Work out the finished part from the listing and answer in its coordinate system (mm). Face numbers are marked on the shaded views. A direction names the side the tool comes from. Coordinates: 2 decimals unless noted, no trailing zeros. Order: outer loops, then holes, each group sorted by start corner. A loop starts at its lowest first (then second) coordinate and runs counter-clockwise, first axis right, second up. Notation, with made-up numbers: (49.5, 8) -> (58.5, 8) arc R28 ccw to (58.5, 42) -> close; hole circle Ø4 at (-8.5, 12.25). An arc over 180 degrees is marked (long way). Write item = value, one per line. Start each with the question number.
Q1. A flat-ended cylindrical pin translates along its axis: pin 1 (3 mm diameter, centred on x = -5.5, y = 1.5, fed in from +Z). Find the tip coordinate at first contact, or state that the pin passes through.
Q2. The part is cut by section D-D, the plane z = 6. Determine the outline of the cut face in (x, y), plus the area to 3 significant figures.
Q3. The part is cut by section A-A, the plane x = 5.5. Determine the outline of the cut face in (y, z).
Q4. Which of the six approach directions +Z, -Z, +X, -X, +Y, -Y give full straight-line access (tool end or side, diameter ignored) to the marked faces 1, 2, 3, 4 and 5?
Q5. The part is cut by section C-C, the plane x = -2. Determine the outline of the cut face in (y, z), plus the area to 3 significant figures.
Q6. Straight lines are drawn through the part: L1, parallel to Z at x = 5.5, y = 0.25; L2, parallel to X at y = -0.6, z = 6; L3, parallel to Z at x = -1.75, y = -2.25. For each, find the intervals that lie inside material, in ascending order. Write a range as from..to.
Q7. The part is cut by section B-B, the plane z = 1.75. Determine the outline of the cut face in (x, y).
```python
from build123d import *

# Parameters (mm, degrees)
SKETCH1_R             = 1.15
BOSS_EXTRUDE1_DEPTH   = 2.6
BOSS_EXTRUDE2_DEPTH   = 4
SKETCH3_W             = 3
SKETCH3_H             = 5.2
BOSS_EXTRUDE3_DEPTH   = 8
BOSS_EXTRUDE4_DEPTH   = 2.6
CHAMFER1_SIZE         = 1
CHAMFER2_SIZE         = 0.75
CHAMFER2_SIZE2        = 1.299038106
CHAMFER2_PART_2_SIZE  = 0.75
CHAMFER2_PART_2_SIZE2 = 1.299038106


with BuildPart() as part:
    # Sketch1 → Boss-Extrude1 (new body, symmetric)
    with BuildSketch(Plane(origin=(0, 0, 0), x_dir=(1, 0, 0), z_dir=(0, 1, 0))):
        Polygon((4, 0), (8, 0), (8, -12), (3, -12), (3, -4), (-8, -4), (-8, 0), (-4, 0), (-4, -2), (4, -2), align=None)
        with Locations((5.5, -6)):
            Circle(SKETCH1_R, mode=Mode.SUBTRACT)
    extrude(amount=BOSS_EXTRUDE1_DEPTH, both=True)

    # Sketch2 → Boss-Extrude2 (add)
    with BuildSketch(Plane.ZY.offset(8)):
        Polygon((-1.5, -1.25), (-1.5, -2.6), (-4.5, -2.6), (-4.5, 2.6), (-1.5, 2.6), (-1.5, 1.25), (0, 1.25), (0, -1.25), align=None)
    boss_extrude2 = extrude(amount=-BOSS_EXTRUDE2_DEPTH)

    # Mirror1: Boss-Extrude2 across plane
    add(boss_extrude2.mirror(Plane(origin=(0, 0, 0), x_dir=(0, 0, 1), z_dir=(1, 0, 0))))

    # Sketch3 → Boss-Extrude3 (add)
    with BuildSketch(Plane(origin=(-4, 0, 0), x_dir=(0, 0, -1), z_dir=(1, 0, 0))):
        with Locations((3, 0)):
            Rectangle(SKETCH3_W, SKETCH3_H)
    extrude(amount=BOSS_EXTRUDE3_DEPTH)

    # Sketch4 → Boss-Extrude4 (add, symmetric)
    with BuildSketch(Plane(origin=(0, 0, 0), x_dir=(1, 0, 0), z_dir=(0, 1, 0))):
        with BuildLine():
            Line((-4, -1), (-4, -2))
            Line((-4, -2), (-3.464101615, -2))
            ThreePointArc((-3.464101615, -2), (-0.63227674, -0.050287843), (2.666666667, -1.01857603))
            ThreePointArc((2.666666667, -1.01857603), (3.372677996, -0.979231367), (3.333333333, -0.273220038))
            ThreePointArc((3.333333333, -0.273220038), (-0.493116, 0.975624243), (-4, -1))
        make_face()
    extrude(amount=BOSS_EXTRUDE4_DEPTH, both=True)

    # Chamfer1
    chamfer1_edges = [part.edges().sort_by_distance(p)[0] for p in [
        (-8, 1.925, 0),
        (8, 1.925, 0),
        (8, 0, 12),
        (3, 0, 12),
        (3, 0, 4),
        (-8, 0, 4),
        (-8, -1.925, 0),
        (0, -2.6, -4.5),
        (0, 2.6, -4.5),
        (-8, 0, -4.5),
        (-8, -2.6, -3),
        (-8, 2.6, -3),
        (8, -1.925, 0),
        (8, 0, -4.5),
        (8, -2.6, -3),
        (8, 2.6, -3),
    ]]
    chamfer(chamfer1_edges, length=CHAMFER1_SIZE)

    # Chamfer2
    chamfer2_edges = [part.edges().sort_by_distance(p)[0] for p in [
        (4.35, -2.6, 6),
    ]]
    chamfer2_side = [part.faces().sort_by_distance(p)[0] for p in [
        (5.5, -2.6, 0.206155281),
    ]]
    chamfer(chamfer2_edges, length=CHAMFER2_SIZE, length2=CHAMFER2_SIZE2, reference=chamfer2_side[0])

    # Chamfer2 part 2
    chamfer2_part_2_edges = [part.edges().sort_by_distance(p)[0] for p in [
        (4.35, 2.6, 6),
    ]]
    chamfer2_part_2_side = [part.faces().sort_by_distance(p)[0] for p in [
        (5.5, 2.6, 0.206155281),
    ]]
    chamfer(chamfer2_part_2_edges, length=CHAMFER2_PART_2_SIZE, length2=CHAMFER2_PART_2_SIZE2, reference=chamfer2_part_2_side[0])


solid = part.part
```
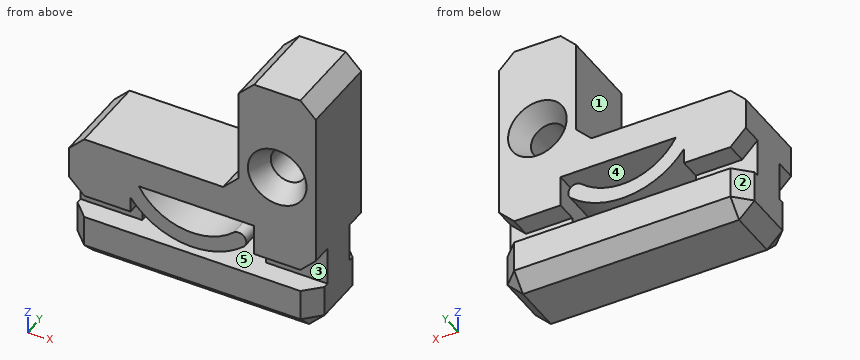
Model answer:
q1.pin_1 = 4
q2.outline = (3, -2.6) -> (3.6, -2.6) -> (4.35, -1.3) -> (4.35, 1.3) -> (3.6, 2.6) -> (3, 2.6) -> close; (6.65, -1.3) -> (7.4, -2.6) -> (8, -2.6) -> (8, 2.6) -> (7.4, 2.6) -> (6.65, 1.3) -> close
q2.area = 12.1 mm2
q3.outline = (-2.6, -3.5) -> (-1.6, -4.5) -> (1.6, -4.5) -> (2.6, -3.5) -> (2.6, -1.5) -> (1.25, -1.5) -> (1.25, 0) -> (2.6, 0) -> (2.6, 4.1) -> (1.3, 4.85) -> (-1.3, 4.85) -> (-2.6, 4.1) -> (-2.6, 0) -> (-1.25, 0) -> (-1.25, -1.5) -> (-2.6, -1.5) -> close; (-2.6, 7.9) -> (-1.3, 7.15) -> (1.3, 7.15) -> (2.6, 7.9) -> (2.6, 12) -> (-2.6, 12) -> close
q4.face_1 = +Z, -X, +Y, -Y
q4.face_2 = -Z, -X, +Y
q4.face_3 = +X, -Y
q4.face_4 = +Y, -Y
q4.face_5 = none
q5.outline = (-2.6, -3.5) -> (-1.6, -4.5) -> (1.6, -4.5) -> (2.6, -3.5) -> (2.6, -1.5) -> (-2.6, -1.5) -> close; (-2.6, -0.58) -> (2.6, -0.58) -> (2.6, 0.54) -> (-2.6, 0.54) -> close; (-2.6, 2) -> (2.6, 2) -> (2.6, 4) -> (-2.6, 4) -> close
q5.area = 30.8 mm2
q6.L1 = -4.5..4.85, 7.15..12
q6.L2 = 3..4.35, 6.65..8
q6.L3 = -3.85..-1.5, -0.68..0.4, 2..4
q7.outline = (-8, -2.6) -> (-3.31, -2.6) -> (-3.31, 2.6) -> (-8, 2.6) -> close; (4, -2.6) -> (8, -2.6) -> (8, 2.6) -> (4, 2.6) -> close
